Can you work these out from the model? Positions are in its coordinate system, mm. Face numbers are marked on the shaded views. Give positions to 0.01 mm unless a question says otherwise; leave off trailing zeros. Order: outer loops, then holes, each group sorted by start corner. A loop starts at its lowest first (then second) coordinate and runs counter-clockwise, first axis right, second up.
Item 1: I want a section at A-A, the plane x = 29. Write out the boundary of the cut face in (y, z), then the cut area to 3 significant figures.
Item 2: I want a section at B-B, the plane y = -6.6. Write out the boundary of the cut face in (x, z).
Item 3: I want a section at D-D, the plane z = 38. Write out the boundary of the cut face in (x, y).
Item 4: I want a section at C-C, the plane x = 4. Write out the boundary of the cut face in (y, z).
Item 5: If we mould it in two halves opening along Y, with no side actions, what happens to the marked faces 1, 2 and 3? For each: +Y half, -Y half, draft (parallel to the pull), parting line (faces both ways), or undercut.
Item 6: I'm going to push flat-ended pins straight in: pin 1 Ø5 at (x, y) = (32.49, -6.6) entering from -Z; pin 2 Ø5.5 at (y, z) = (-5, 52.5) entering from -X; pin 3 Ø1 at (y, z) = (-7.5, 43.5) entering from +X; pin 4 Ø1 at (y, z) = (-11.5, 17.5) entering from -X. Where does each tip first touch, or does it pass through?
Item 7: If I drill on line 1 along Y through (x, z) = (15, 31.5); line 2 along X through (y, z) = (-6.6, 53.2); line 3 along X through (y, z) = (-6.6, 2), over which ranges is the centre line in solid material (lowest first)?
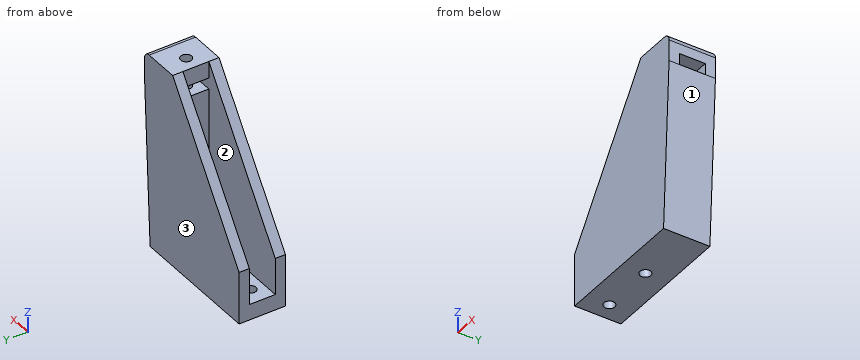
```python
from build123d import *

# Parameters (mm, degrees)
PAD034_DEPTH    = 13.2
SKETCH109_R     = 1.55
POCKET067_DEPTH = 80
SKETCH110_W     = 28.3584052975
SKETCH110_H     = 7.4
POCKET068_DEPTH = 51
SKETCH112_R     = 1.55
POCKET069_DEPTH = 10
FILLET_R        = 2
SKETCH113_W     = 3.2
SKETCH113_H     = 7.4
POCKET070_DEPTH = 12


with BuildPart() as part:
    # Sketch108 → Pad034 (new body)
    with BuildSketch(Plane.XZ):
        Polygon((40.3584052975, 55.5), (40.3584052975, 47.5), (38, 0), (0, 0), (0, 15), (28.3584052975, 55.5), align=None)
    extrude(amount=PAD034_DEPTH)

    # Sketch109 (on Face3 of Pad034) → Pocket067 (cut)
    with BuildSketch(Plane(origin=(0, 0, 0), x_dir=(1, 0, 0), z_dir=(0, 0, -1))):
        with Locations((4.9809052975, 6.6)):
            Circle(SKETCH109_R)
        with Locations((20.3584052975, 6.6)):
            Circle(SKETCH109_R)
    extrude(amount=-POCKET067_DEPTH, mode=Mode.SUBTRACT)

    # Sketch110 (on Face2 of Pocket067) → Pocket068 (cut)
    with BuildSketch(Plane(origin=(0, 0, 55.5), x_dir=(-1, 0, 0), z_dir=(0, 0, 1))):
        with Locations((-14.1792026487, 6.6)):
            Rectangle(SKETCH110_W, SKETCH110_H)
    extrude(amount=-POCKET068_DEPTH, mode=Mode.SUBTRACT)

    # Sketch112 (on Face2 of Pocket068) → Pocket069 (cut)
    with BuildSketch(Plane(origin=(0, 0, 55.5), x_dir=(-1, 0, 0), z_dir=(0, 0, 1))):
        with Locations((-32.4934052975, 6.6)):
            Circle(SKETCH112_R)
    extrude(amount=-POCKET069_DEPTH, mode=Mode.SUBTRACT)

    # Fillet
    fillet_edges = [part.edges().sort_by_distance(p)[0] for p in [
        (40.358405, -6.6, 55.5),
    ]]
    fillet(fillet_edges, radius=FILLET_R)

    # Sketch113 (on Face1 of Fillet) → Pocket070 (cut)
    with BuildSketch(Plane(origin=(40.3584052975, 0, 0), x_dir=(0, 0, 1), z_dir=(1, 0, 0))):
        with Locations((49.1, 6.6)):
            Rectangle(SKETCH113_W, SKETCH113_H)
    extrude(amount=-POCKET070_DEPTH, mode=Mode.SUBTRACT)


solid = part.part
```
Results list:
1. outline: (-13.2, 0) - (0, 0) - (0, 55.5) - (-13.2, 55.5) - close; hole (-10.3, 47.5) - (-2.9, 47.5) - (-2.9, 50.7) - (-10.3, 50.7) - close
1. area: 709 mm2
2. outline: (0, 0) - (3.43, 0) - (3.43, 4.5) - (0, 4.5) - close; (6.53, 0) - (18.81, 0) - (18.81, 4.5) - (6.53, 4.5) - close; (21.91, 0) - (38, 0) - (40.36, 47.5) - (34.04, 47.5) - (34.04, 45.5) - (30.94, 45.5) - (30.94, 47.5) - (28.36, 47.5) - (28.36, 4.5) - (21.91, 4.5) - close; (28.36, 50.7) - (30.94, 50.7) - (30.94, 55.5) - (28.36, 55.5) - close; (34.04, 50.7) - (40.36, 50.7) - (40.36, 53.5) arc R2 ccw to (38.36, 55.5) - (34.04, 55.5) - close
3. outline: (16.1, -13.2) - (39.89, -13.2) - (39.89, 0) - (16.1, 0) - (16.1, -2.9) - (28.36, -2.9) - (28.36, -10.3) - (16.1, -10.3) - close
4. outline: (-13.2, 0) - (-7.8, 0) - (-7.8, 4.5) - (-10.3, 4.5) - (-10.3, 20.71) - (-13.2, 20.71) - close; (-5.4, 0) - (0, 0) - (0, 20.71) - (-2.9, 20.71) - (-2.9, 4.5) - (-5.4, 4.5) - close
5. face 1: draft
5. face 2: undercut
5. face 3: +Y half
6. pin 1: stops at z = 0
6. pin 2: stops at x = 25.01
6. pin 3: stops at x = 40.18
6. pin 4: stops at x = 1.4
7. line 1: y = -13.2 to -10.3, -2.9 to 0
7. line 2: x = 28.36 to 30.94, 34.04 to 40.36
7. line 3: x = 0 to 3.43, 6.53 to 18.81, 21.91 to 38.1
